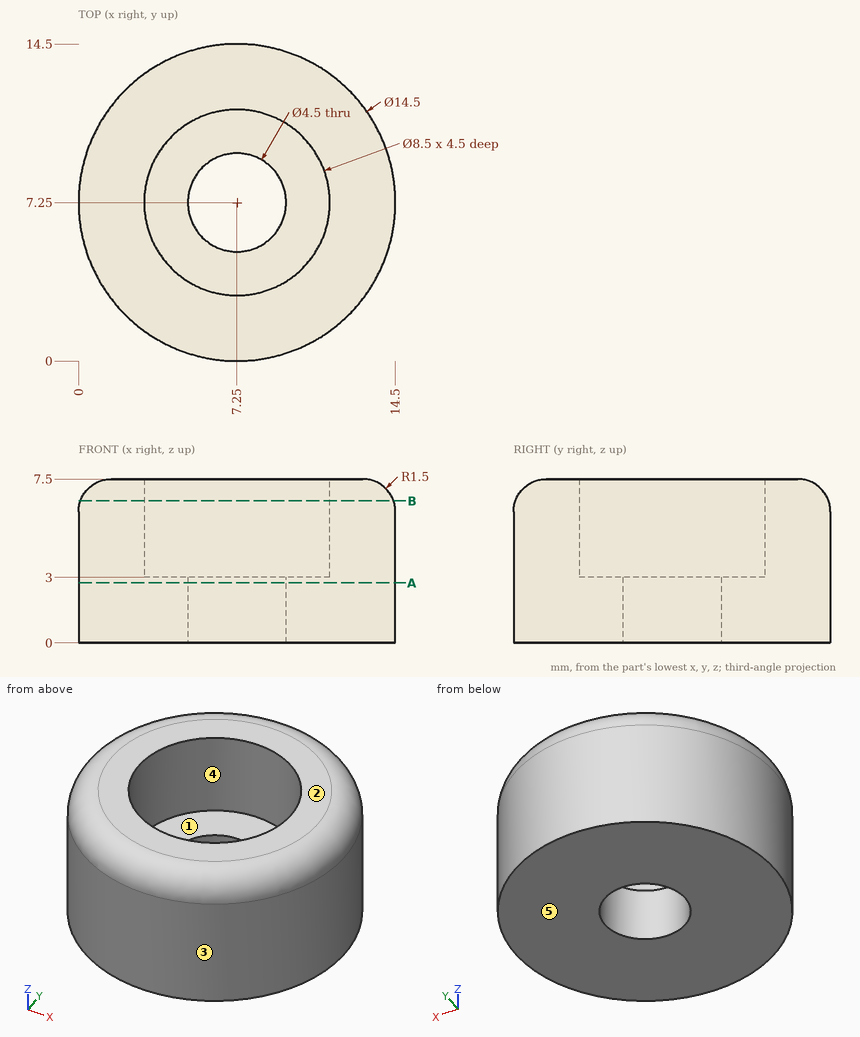
Input: dimensioned drawing with shaded views. Units: mm. Origin: part minimum x, y, z. A direction names the side the tool comes from. Round coordinates to 2 decimals unless told otherwise and drop trailing zeros. Loops run counter-clockwise (first coordinate to the right, second up) from the corner with the lowest first, then second, coordinate; pieces in that order, holes last. Notation, with made-up numbers: (-16.75, -24.5) -> (10.25, -24.5) arc R19 ccw to (10.25, -12.5) -> close; hole circle Ø3 at (33, 24.25). An arc over 180 degrees is marked (long way). One line per item, written item: value.
(1) Mould query, pull axis Y, two halves, no side actions, for the marked faces 3, 4 and 5. Classes: pulls with the +Y half, pulls with the -Y half, needs draft (parallel to the pull), parting line crosses it, or undercut.
Geometry check:
face 3: parting line crosses it
face 4: undercut
face 5: needs draft
(2) Set-up query: the marked faces 1 and 2. Return all of +Z, -Z, +X, -X, +Y, -Y with unobstructed straight access to the full face (end or side cutting, diameter ignored); none if empty.
Geometry check:
face 1: +Z
face 2: +Z, +X, -X, +Y, -Y
(3) Section B-B (z = 6.5). Return the cut outline in (x, y).
Geometry check:
outline: circle Ø14.33 at (7.25, 7.25); hole circle Ø8.5 at (7.25, 7.25)
(4) Section A-A (z = 2.75). Return the cut outline in (x, y), plus the area to 3 significant figures.
Geometry check:
outline: circle Ø14.5 at (7.25, 7.25); hole circle Ø4.5 at (7.25, 7.25)
area: 149 mm2
(5) Material intervals for line 1 (Y direction, x = 7.25, z = 1.5); line 2 (Z direction, x = 6.5, y = 11.25); line 3 (Y direction, x = 7.25, z = 5.05), sorted ascending. Write a range as [from, to].
Geometry check:
line 1: [0, 5], [9.5, 14.5]
line 2: [0, 3]
line 3: [0, 3], [11.5, 14.5]
(6) Pin query (flat end, axial travel): pin 1 (3.5 mm diameter, centred on x = 7.25, y = 7.25, fed in from -Z); pin 2 (1.5 mm diameter, centred on x = 10.5, z = 2, fed in from +Y); pin 3 (4 mm diameter, centred on x = 4, z = 6, fed in from +Y); pin 4 (4 mm diameter, centred on x = 6.5, y = 6, fed in from +Z). Return the tip coordinate at first contact, or that it passes through.
Geometry check:
pin 1: through
pin 2: y = 14.06
pin 3: y = 14.39
pin 4: z = 3
